Check sheet for the modelled part. Datum: model origin and axes. Units: mm. Give positions to 0.01 mm unless a question says otherwise; leave off trailing zeros. Order: outer loops, then holes, each group sorted by start corner. A loop starts at its lowest first (then second) coordinate and runs counter-clockwise, first axis right, second up. Notation, with made-up numbers: (-24.75, -38) -> (-19.75, -38) arc R19 ccw to (-19.75, -10) -> close; hole circle Ø1 at (76.5, 7.25). An arc over 180 degrees is marked (long way). Answer in a Markdown table with one row per item. Add a question column.
(1) Go/stop test with a flat-tipped pin: pin 1 (1.5 mm diameter, centred on x = -1, y = 1, fed in from +Z). Record where the tip stops, or that it passes through.
(2) Cross-section at A-A (y = 7.75). Record the cut outline in (x, z), then the cut area to 3 significant figures.
(3) Release check for a two-part mould opening along Z. For faces 1 (the face through (2.312, 4.555, 0.513)), 2 (the face through (-0.245, 3.863, 1.103)), 3 (the face through (0, 9.525, 0)), 4 (the face through (0.043, 8.181, 0.192)) record: released by +Z, released by -Z, zero draft, split by the parting line, or undercut.
(4) Thickness scan on L1, parallel to Z at x = -0.05, y = 1.25; L2, parallel to Y at x = 1.3, z = 1. Record the ranges inside material, lowest first. Write a range as [from, to].
(5) Cross-section at B-B (y = 1). Record the cut outline in (x, z).
```python
from build123d import *

# Parameters (mm, degrees)
CHAMFER1_SIZE             = 0.254
F_4_40_TAPPED_HOLE1_D     = 2.2606
F_4_40_TAPPED_HOLE1_DEPTH = 7.62
F_4_40_TAPPED_HOLE1_TIP   = 0.679152758


with BuildPart() as part:
    # Sketch1 → Revolve1 (revolve)
    with BuildSketch(Plane.XY, mode=Mode.PRIVATE) as revolve1_sk:
        with BuildLine():
            Line((0, 0), (-2.36855, 0))
            Line((-2.36855, 0), (-2.36855, 8.7376))
            ThreePointArc((-2.36855, 8.7376), (-2.13792588, 9.29437588), (-1.58115, 9.525))
            Line((-1.58115, 9.525), (0, 9.525))
            Line((0, 9.525), (0, 0))
        make_face()
    revolve(revolve1_sk.sketch.rotate(Axis((0, 0, 0), (0, 1, 0)), 270), axis=Axis((0, 0, 0), (0, 1, 0)))

    # Chamfer1
    chamfer1_edges = [part.edges().sort_by_distance(p)[0] for p in [
        (0, 0, 2.36855),
    ]]
    chamfer(chamfer1_edges, length=CHAMFER1_SIZE)

    # 4-40 Tapped Hole1
    with Locations(Plane(origin=(0, 0, 0), x_dir=(-1, 0, 0), z_dir=(0, -1, 0))):
        with Locations((0, 0)):
            Hole(F_4_40_TAPPED_HOLE1_D / 2, depth=F_4_40_TAPPED_HOLE1_DEPTH)
            with Locations((0, 0, -(F_4_40_TAPPED_HOLE1_DEPTH + F_4_40_TAPPED_HOLE1_TIP / 2))):  # 118° drill point
                Cone(0, F_4_40_TAPPED_HOLE1_D / 2, F_4_40_TAPPED_HOLE1_TIP, mode=Mode.SUBTRACT)


solid = part.part
```
Answer below:
| question | item | result |
|---|---|---|
| 1 | pin 1 | stops at z = 2.36 |
| 2 | outline | circle Ø4.74 at (0, 0); hole circle Ø1.83 at (0, 0) |
| 2 | area | 15.0 mm² |
| 3 | face 1 | split by the parting line |
| 3 | face 2 | undercut |
| 3 | face 3 | zero draft |
| 3 | face 4 | undercut |
| 4 | L1 | z = [-2.37, -1.13], [1.13, 2.37] |
| 4 | L2 | y = [0, 9.52] |
| 5 | outline | circle Ø4.74 at (0, 0); hole circle Ø2.26 at (0, 0) |
